Can you work these out from the model? Positions are in its coordinate system, mm. A direction names the side the tool comes from. Coordinates: 2 decimals unless noted, no trailing zeros. Order: outer loops, then holes, each group sorted by start corner. A loop starts at its lowest first (then second) coordinate and runs counter-clockwise, first axis right, second up. Notation, with made-up numbers: M 2,43 L 8,43 A13 ccw 8,62 Z; hole C -35,-37 d8. An arc over 180 degrees is marked long. Answer as a JSON object with one key per item and string values.
from build123d import *

# Parameters (mm, degrees)
V3_BOX_FOOTPRINT_100_X_45_MM_W                 = 100
V3_BOX_FOOTPRINT_100_X_45_MM_H                 = 45
V3_BOX_HEIGHT_35_MM_DEPTH                      = 35
V3_REAR_OPENING_96_X_31_MM_W                   = 96
V3_REAR_OPENING_96_X_31_MM_H                   = 31
V3_CAVITY_ALL_WALLS_2_MM_DEPTH                 = 43
V3_SQUARE_BEAMS_10_X_10_PITCH_95_MM_W          = 10
V3_SQUARE_BEAMS_10_X_10_PITCH_95_MM_H          = 10
V3_FORWARD_BEAM_LENGTH_65_MM_DEPTH             = 65
V3_LEFT_PCB_EAR_PROFILE_W                      = 10
V3_LEFT_PCB_EAR_PROFILE_H                      = 10
V3_LEFT_INWARD_EAR_5_MM_DEPTH                  = 5
V3_RIGHT_PCB_EAR_PROFILE_W                     = 10
V3_RIGHT_PCB_EAR_PROFILE_H                     = 10
V3_RIGHT_INWARD_EAR_5_MM_DEPTH                 = 5
V3_PCB_ROOF_PAIR_PITCH_85_MM_R                 = 1.7
V3_M3_ROOF_HOLES_DIAMETER_3_4_MM_DEPTH         = 2
V3_PCB_FORWARD_PAIR_ROW_SPACING_60_MM_R        = 1.7
V3_M3_PCB_EAR_HOLES_DEPTH                      = 10
V3_CHASSIS_TOP_HOLES_WIDTH_95_DEPTH_40_M_R     = 1.7
V3_M3_BEAM_TOP_BOTTOM_HOLES_DEPTH              = 10
V3_HANGING_PLATE_OFFSET_26_THICKNESS_2_5_W     = 110
V3_HANGING_PLATE_OFFSET_26_THICKNESS_2_5_H     = 2.5
V3_MOUNTING_PLATE_DOWNWARD_15_MM_WIDTH_1_DEPTH = 15
FOUR_HORIZONTAL_SLOTS_3_4_X_5_4_MM_DEPTH       = 2.5
CUT_EXTRUDE_1_DEPTH                            = 93.059763198


with BuildPart() as part:
    # V3 box footprint 100 x 45 mm → V3 box height 35 mm (new body)
    with BuildSketch(Plane.XY):
        with Locations((0, 22.5)):
            Rectangle(V3_BOX_FOOTPRINT_100_X_45_MM_W, V3_BOX_FOOTPRINT_100_X_45_MM_H)
    extrude(amount=V3_BOX_HEIGHT_35_MM_DEPTH)

    # V3 rear opening 96 x 31 mm → V3 cavity all walls 2 mm (cut)
    with BuildSketch(Plane(origin=(0, 45, 0), x_dir=(1, 0, 0), z_dir=(0, 1, 0))):
        with Locations((0, -17.5)):
            Rectangle(V3_REAR_OPENING_96_X_31_MM_W, V3_REAR_OPENING_96_X_31_MM_H)
    extrude(amount=-V3_CAVITY_ALL_WALLS_2_MM_DEPTH, mode=Mode.SUBTRACT)

    # V3 square beams 10 x 10 pitch 95 mm → V3 forward beam length 65 mm (add)
    with BuildSketch(Plane.XZ):
        with Locations((-47.5, 30)):
            Rectangle(V3_SQUARE_BEAMS_10_X_10_PITCH_95_MM_W, V3_SQUARE_BEAMS_10_X_10_PITCH_95_MM_H)
        with Locations((47.5, 30)):
            Rectangle(V3_SQUARE_BEAMS_10_X_10_PITCH_95_MM_W, V3_SQUARE_BEAMS_10_X_10_PITCH_95_MM_H)
    extrude(amount=V3_FORWARD_BEAM_LENGTH_65_MM_DEPTH)

    # V3 left PCB ear profile → V3 left inward ear 5 mm (add)
    with BuildSketch(Plane(origin=(-42.5, 0, 0), x_dir=(0, 0, -1), z_dir=(1, 0, 0))):
        with Locations((-30, -20)):
            Rectangle(V3_LEFT_PCB_EAR_PROFILE_W, V3_LEFT_PCB_EAR_PROFILE_H)
    extrude(amount=V3_LEFT_INWARD_EAR_5_MM_DEPTH)

    # V3 right PCB ear profile → V3 right inward ear 5 mm (add)
    with BuildSketch(Plane.ZY.offset(-42.5)):
        with Locations((30, -20)):
            Rectangle(V3_RIGHT_PCB_EAR_PROFILE_W, V3_RIGHT_PCB_EAR_PROFILE_H)
    extrude(amount=V3_RIGHT_INWARD_EAR_5_MM_DEPTH)

    # V3 PCB roof pair pitch 85 mm → V3 M3 roof holes diameter 3.4 mm (cut)
    with BuildSketch(Plane.XY.offset(35)):
        with Locations((-42.5, 40)):
            Circle(V3_PCB_ROOF_PAIR_PITCH_85_MM_R)
        with Locations((42.5, 40)):
            Circle(V3_PCB_ROOF_PAIR_PITCH_85_MM_R)
    extrude(amount=-V3_M3_ROOF_HOLES_DIAMETER_3_4_MM_DEPTH, mode=Mode.SUBTRACT)

    # V3 PCB forward pair row spacing 60 mm → V3 M3 PCB ear holes (cut)
    with BuildSketch(Plane.XY.offset(35)):
        with Locations((-42.5, -20)):
            Circle(V3_PCB_FORWARD_PAIR_ROW_SPACING_60_MM_R)
        with Locations((42.5, -20)):
            Circle(V3_PCB_FORWARD_PAIR_ROW_SPACING_60_MM_R)
    extrude(amount=-V3_M3_PCB_EAR_HOLES_DEPTH, mode=Mode.SUBTRACT)

    # V3 chassis top holes width 95 depth 40 mm → V3 M3 beam top bottom holes (cut)
    with BuildSketch(Plane.XY.offset(35)):
        with Locations((-47.5, -55)):
            Circle(V3_CHASSIS_TOP_HOLES_WIDTH_95_DEPTH_40_M_R)
        with Locations((-47.5, -15)):
            Circle(V3_CHASSIS_TOP_HOLES_WIDTH_95_DEPTH_40_M_R)
        with Locations((47.5, -55)):
            Circle(V3_CHASSIS_TOP_HOLES_WIDTH_95_DEPTH_40_M_R)
        with Locations((47.5, -15)):
            Circle(V3_CHASSIS_TOP_HOLES_WIDTH_95_DEPTH_40_M_R)
    extrude(amount=-V3_M3_BEAM_TOP_BOTTOM_HOLES_DEPTH, mode=Mode.SUBTRACT)

    # V3 hanging plate offset 26 thickness 2.5 mm → V3 mounting plate downward 15 mm width 110 (add)
    with BuildSketch(Plane(origin=(0, 0, 25), x_dir=(-1, 0, 0), z_dir=(0, 0, -1))):
        with Locations((0, -27.25)):
            Rectangle(V3_HANGING_PLATE_OFFSET_26_THICKNESS_2_5_W, V3_HANGING_PLATE_OFFSET_26_THICKNESS_2_5_H)
    extrude(amount=V3_MOUNTING_PLATE_DOWNWARD_15_MM_WIDTH_1_DEPTH)

    # V3 slots 6 mm below beam underside centers 20 and 47.5 → Four horizontal slots 3.4 x 5.4 mm (cut)
    with BuildSketch(Plane.XZ.offset(28.5)):
        with BuildLine():
            Line((-48.5, 20.7), (-46.5, 20.7))
            ThreePointArc((-46.5, 20.7), (-44.8, 19), (-46.5, 17.3))
            Line((-46.5, 17.3), (-48.5, 17.3))
            ThreePointArc((-48.5, 17.3), (-50.2, 19), (-48.5, 20.7))
        make_face()
        with BuildLine():
            Line((-21, 20.7), (-19, 20.7))
            ThreePointArc((-19, 20.7), (-17.3, 19), (-19, 17.3))
            Line((-19, 17.3), (-21, 17.3))
            ThreePointArc((-21, 17.3), (-22.7, 19), (-21, 20.7))
        make_face()
        with BuildLine():
            Line((19, 20.7), (21, 20.7))
            ThreePointArc((21, 20.7), (22.7, 19), (21, 17.3))
            Line((21, 17.3), (19, 17.3))
            ThreePointArc((19, 17.3), (17.3, 19), (19, 20.7))
        make_face()
        with BuildLine():
            Line((46.5, 20.7), (48.5, 20.7))
            ThreePointArc((48.5, 20.7), (50.2, 19), (48.5, 17.3))
            Line((48.5, 17.3), (46.5, 17.3))
            ThreePointArc((46.5, 17.3), (44.8, 19), (46.5, 20.7))
        make_face()
    extrude(amount=-FOUR_HORIZONTAL_SLOTS_3_4_X_5_4_MM_DEPTH, mode=Mode.SUBTRACT)

    # 草图2 → 切除-拉伸1 (cut, through all)
    with BuildSketch(Plane(origin=(0, 0, 0), x_dir=(-1, 0, 0), z_dir=(0, 0, -1))):
        with BuildLine():
            Line((-32.029979042, 6.459471041), (-21.029979042, 6.459471041))
            ThreePointArc((-21.029979042, 6.459471041), (-19.570508001, 5), (-21.029979042, 3.540528959))
            Line((-21.029979042, 3.540528959), (-32.029979042, 3.540528959))
            ThreePointArc((-32.029979042, 3.540528959), (-33.489450083, 5), (-32.029979042, 6.459471041))
        make_face()
        with BuildLine():
            Line((23.620107008, 6.558669056), (34.620107008, 6.558669056))
            ThreePointArc((34.620107008, 6.558669056), (36.178776063, 5), (34.620107008, 3.441330944))
            Line((34.620107008, 3.441330944), (23.620107008, 3.441330944))
            ThreePointArc((23.620107008, 3.441330944), (22.061437952, 5), (23.620107008, 6.558669056))
        make_face()
    extrude(amount=-CUT_EXTRUDE_1_DEPTH, mode=Mode.SUBTRACT)


solid = part.part
Item 1: I want a section at D-D, the plane z = 6.5. Write out the boundary of the cut face in (x, y).
Answers follow:
{"outline": "M -50,0 L 50,0 L 50,45 L 48,45 L 48,2 L -48,2 L -48,45 L -50,45 Z"}
Item 2: I want a section at C-C, the plane y = 29.5. Write out the boundary of the cut face in (x, z), plus the area to 3 significant figures.
Answers follow:
{"outline": "M -50,0 L 50,0 L 50,35 L -50,35 Z; hole M -48,2 L 48,2 L 48,33 L -48,33 Z", "area": "524 mm^2"}
Item 3: I want a section at A-A, the plane z = 19. Write out the boundary of the cut face in (x, y).
Answers follow:
{"outline": "M -55,-28.5 L -50.2,-28.5 L -50.2,-26 L -55,-26 Z; M -50,0 L 50,0 L 50,45 L 48,45 L 48,2 L -48,2 L -48,45 L -50,45 Z; M -44.8,-28.5 L -22.7,-28.5 L -22.7,-26 L -44.8,-26 Z; M -17.3,-28.5 L 17.3,-28.5 L 17.3,-26 L -17.3,-26 Z; M 22.7,-28.5 L 44.8,-28.5 L 44.8,-26 L 22.7,-26 Z; M 50.2,-28.5 L 55,-28.5 L 55,-26 L 50.2,-26 Z"}
Item 4: Which directions (+Z, -Z, +X, -X, +Y, -Y) give clear straight access to the entire face, cutting with the end or side of a thin tool? Please do faces 4 (the flat face through (1, -28.5, 18)), 5 (the cylindrical face through (-50.2, -27.3, 19)), 6 (the flat face through (54, -27, 25)), 7 (the flat face through (-42.5, -7, 30)), 8 (the flat face through (-48, 24, 18)).
Answers follow:
{"face 4": "-Z, +X, -X, -Y", "face 5": "-Y", "face 6": "+Z, +X, +Y, -Y", "face 7": "+Z, -Z", "face 8": "+Y"}
Item 5: I want a section at B-B, the plane y = -55. Write out the boundary of the cut face in (x, z).
Answers follow:
{"outline": "M -52.5,25 L -49.2,25 L -49.2,35 L -52.5,35 Z; M -45.8,25 L -42.5,25 L -42.5,35 L -45.8,35 Z; M 42.5,25 L 45.8,25 L 45.8,35 L 42.5,35 Z; M 49.2,25 L 52.5,25 L 52.5,35 L 49.2,35 Z"}
Item 6: Please list where these lines run through material, in increasing order: line 1 (Y direction, x = -47.5, z = 28); line 2 (X direction, y = -5, z = 33.5); line 3 (X direction, y = 26.5, z = 25.5).
Answers follow:
{"line 1": "y = -65 to -56.7, -53.3 to -16.7, -13.3 to 2", "line 2": "x = -52.5 to -42.5, 42.5 to 52.5", "line 3": "x = -50 to -48, 48 to 50"}
Item 7: I'm going to push flat-ended pins straight in: pin 1 (6 mm diameter, centred on y = -24, z = 30, fed in from -X); pin 2 (9.5 mm diameter, centred on y = 20, z = 11.5, fed in from -X); pin 3 (16.5 mm diameter, centred on x = 0.5, z = 17, fed in from -Y). Where does each tip first touch, or does it pass through?
Answers follow:
{"pin 1": "stops at x = -52.5", "pin 2": "stops at x = -50", "pin 3": "stops at y = -28.5"}
Item 8: If we mould it in two halves opening along X, with no side actions, what happens to faces 1 (the flat face through (51, 0, 30)), 2 (the flat face through (-42.5, -45, 30)), 3 (the flat face through (-52.5, -32, 30))? For each: pulls with the +X half, pulls with the -X half, needs draft (parallel to the pull), parting line crosses it, or undercut.
Answers follow:
{"face 1": "needs draft", "face 2": "undercut", "face 3": "pulls with the -X half"}
